Autodesk Inventor part; units mm, degrees
ref_plane "YZ Plane" through (0, 0, 0) normal (1, 0, 0) x (0, 1, 0)
ref_plane "XZ Plane" through (0, 0, 0) normal (0, 1, 0) x (-1, 0, 0)
ref_plane "XY Plane" through (0, 0, 0) normal (0, 0, 1) x (1, 0, 0)
sketch "Sketch1" plane through (0, 0, 0) normal (0, 0, 1) x (1, 0, 0)
  line L0 (0, 18.05) -> (16, 18.05)
  line L1 (16, 18.05) -> (16, -18.05)
  line L2 (16, -18.05) -> (0, -18.05)
  arc A0 (0, -8.15) -> (0, 8.15) centre (0, 0) ccw
  line L3 (0, -18.05) -> (0, -8.15)
  line L4 (0, 8.15) -> (0, 18.05)
  point P0 (16, 0)
  dimension "d0" = 16.3
  dimension "d1" = 36.1
  dimension "d3" = 16
extrude "Extrusion1" add sketch "Sketch1" along normal mid plane 5
sketch "Sketch2" plane through (0, 0, 2.5) normal (0, 0, 1) x (1, 0, 0)
  arc A0 (0, -6.25) -> (0, 6.25) centre (0, 0) ccw
  arc A1 (0, -8.15) -> (0, 8.15) centre (0, 0) ccw
  line L0 (0, 6.25) -> (0, 8.15)
  line L1 (0, -6.25) -> (0, -8.15)
  dimension "d6" = 12.5
extrude "Extrusion2" add sketch "Sketch2" along normal blind 3.8 and the other way blind 1.8
sketch "Sketch3" plane through (0, 0, 6.3) normal (0, 0, 1) x (1, 0, 0)
  arc A0 (0, -8.15) -> (0, 8.15) centre (0, 0) ccw
  arc A1 (0, -11.15) -> (0, 11.15) centre (0, 0) ccw
  line L0 (0, -8.15) -> (0, -11.15)
  line L1 (0, 8.15) -> (0, 11.15)
  dimension "d11" = 3
extrude "Extrusion3" add sketch "Sketch3" along normal blind 4
sketch "Sketch4" plane through (0, 0, 6.3) normal (0, 0, -1) x (-1, 0, 0)
  arc A0 (0, 8.15) -> (0, -8.15) centre (0, 0) ccw
  line L0 (0, 11.15) -> (0, 8.15)
  arc A1 (0, 11.15) -> (0, -11.15) centre (0, 0) ccw
  line L1 (0, -8.15) -> (0, -11.15)
extrude "Extrusion4" add sketch "Sketch4" along normal up to surface (3.8 mm away)
sketch "Sketch5" plane through (0, 0, 2.5) normal (0, 0, 1) x (1, 0, 0)
  arc A0 (0, -11.15) -> (0, 11.15) centre (0, 0) ccw
  line L0 (16, 18.05) -> (0, 18.05)
  line L1 (3, 18.05) -> (3, 10.7388)
  arc A1 (0, -11.15) -> (0, 11.15) centre (0, 0) ccw
  line L2 (3, -10.7388) -> (3, -18.05)
  line L3 (0, -18.05) -> (16, -18.05)
  line L4 (0, 18.05) -> (0, 11.15)
  line L5 (0, -11.15) -> (0, -18.05)
  dimension "d16" = 3
extrude "Extrusion5" add sketch "Sketch5" along normal up to surface (7.8 mm away)
chamfer "Chamfer1" distance 5 angle 45 1 edges at (11.15, 0, 2.5)
fillet "Fillet1" radius 3 3 edges at (11.7041, -11.1281, 2.5) (11.15, 0, 7.5) (11.7041, 11.1281, 2.5)
sketch "Sketch6" plane through (3, -18.05, 2.5) normal (1, 0, 0) x (0, 0, -1)
  circle A0 centre (-3.8, 32.1) radius 1.6
  circle A1 centre (-3.8, 4) radius 1.6
  line L0 (0, 0) -> (-7.8, 0)
  line L1 (-7.8, 7.3112) -> (-7.8, 0)
  line L2 (0, 36.1) -> (-7.8, 36.1)
  point P0 (2.5, 18.05)
  dimension "d19" = 3.2
  dimension "d20" = 4
  dimension "d21" = 4
  dimension "d22" = 4
extrude "Extrusion6" cut sketch "Sketch6" against normal up to next
fillet "Fillet2" radius 4 2 edges at (1.5, -18.05, 10.3) (1.5, 18.05, 10.3)
fillet "Fillet3" radius 4 2 edges at (16, -18.05, 0) (16, 18.05, 0)
sketch "Sketch7" plane through (3, -18.05, 2.5) normal (1, 0, 0) x (0, 0, -1)
  arc A0 (-3.2482, 5.5018) -> (-2.2844, 4.5129) centre (-3.8, 4) ccw
  arc A1 (-2.2844, 31.5871) -> (-3.2482, 30.5982) centre (-3.8, 32.1) ccw
  circle A2 centre (-3.8, 4) radius 3.5
  circle A3 centre (-3.8, 32.1) radius 3.5
  point P0 (2.5, 18.05)
  dimension "d31" = 7
extrude "Extrusion7" cut sketch "Sketch7" along normal through all
properties part number "x-carriage-holder"
Read the model definition and answer for the solid it produces. Units are mm, in the model's axes. A direction names the side the tool comes from. Give positions to 0.01 mm unless a question says otherwise; leave off trailing zeros. Write each loop counter-clockwise with the first axis right and the second up, starting at its lowest first coordinate (ties: lowest second). Pieces come first, ordered by that corner, then holes. Notation, with made-up numbers: (36, -11) - (80, -11) arc R8 cw to (80, -6) - close; hole circle Ø7 at (30, 62). An arc over 180 degrees is marked (long way). Return JSON: item names as keys, results as strings.
Q1. For a pull along Y with two mould halves and no side action, classify faces 6 (the face through (12, -15, 2.5)), 7 (the face through (1, 17, 9)), 8 (the face through (5.4, -11.5, 3.9)), 9 (the face through (6.25, 0.14, 3.46)) as released by +Y, released by -Y, zero draft, split by the parting line, or undercut.
Reply:
{"face 6": "zero draft", "face 7": "released by +Y", "face 8": "undercut", "face 9": "undercut"}
Q2. A cutting plane is placed at C-C, the plane x = 2.5. Determine the outline of the cut face in (y, z).
Reply:
{"outline": "(-18.05, -2.5) - (-7.76, -2.5) - (-7.76, 0.7) - (-5.73, 0.7) - (-5.73, 6.3) - (-7.76, 6.3) - (-7.76, 10.3) - (-14.05, 10.3) arc R4 ccw to (-18.05, 6.3) - close; (5.73, 0.7) - (7.76, 0.7) - (7.76, -2.5) - (18.05, -2.5) - (18.05, 6.3) arc R4 ccw to (14.05, 10.3) - (7.76, 10.3) - (7.76, 6.3) - (5.73, 6.3) - close; hole circle Ø3.2 at (-14.05, 6.3); hole circle Ø3.2 at (14.05, 6.3)"}
Q3. A cutting plane is placed at D-D, the plane z = 2. Determine the outline of the cut face in (x, y), and give its area (3 significant figures).
Reply:
{"outline": "(0, -18.05) - (12, -18.05) arc R4 ccw to (16, -14.05) - (16, 14.05) arc R4 ccw to (12, 18.05) - (0, 18.05) - (0, 6.25) arc R6.25 cw to (0, -6.25) - close", "area": "509 mm²"}
Q4. Consider line 1 along Z through (x, y) = (1.3, -14.05); line 2 along Y through (x, z) = (4, 0.75); line 3 along X through (y, z) = (11.5, 4). Determine where each line is inside the solid, lowest interval first. Write a range as [from, to].
Reply:
{"line 1": "[-2.5, 4.7], [7.9, 10.3]", "line 2": "[-18.05, -4.8], [4.8, 18.05]", "line 3": "[0, 3]"}
Q5. A cutting plane is placed at B-B, the plane y = 0. Determine the outline of the cut face in (x, z), and give its area (3 significant figures).
Reply:
{"outline": "(6.25, 0.7) - (8.15, 0.7) - (8.15, -2.5) - (16, -2.5) - (16, 2.84) arc R3 cw to (15.27, 3.38) - (12.03, 6.62) arc R3 cw to (11.15, 8.74) - (11.15, 10.3) - (8.15, 10.3) - (8.15, 6.3) - (6.25, 6.3) - close", "area": "86.0 mm²"}
Q6. A cutting plane is placed at A-A, the plane z = 7. Determine the outline of the cut face in (x, y), and give its area (3 significant figures).
Reply:
{"outline": "(0, -17.99) - (3, -17.99) - (3, -15.49) - (0, -15.49) - close; (0, -12.61) - (3, -12.61) - (3, -10.62) - (4.93, -10.62) arc R11.71 ccw to (4.93, 10.62) - (3, 10.62) - (3, 12.61) - (0, 12.61) - (0, 8.15) arc R8.15 cw to (0, -8.15) - close; (0, 15.49) - (3, 15.49) - (3, 17.99) - (0, 17.99) - close", "area": "131 mm²"}
Q7. Given P1, Ø3.5, axis at x = 7, y = 15, coming from the +Z side; P2, Ø3.5, axis at x = 12.5, y = -11.5, coming from the +Z side; P3, Ø5, axis at x = 13.5, y = -6.5, coming from the +Z side; P4, Ø2.5, axis at y = 14.05, z = 6.3, coming from the -X side, each flat-ended and moving along its own axis, determine where each tip first touches the part or whether it passes through.
Reply:
{"P1": "z = 2.92", "P2": "z = 3.41", "P3": "z = 6.17", "P4": "through"}
Q8. For faces 1 (the face through (11.15, -0.2, 9.53)), 2 (the face through (8.15, 0.18, 8.27)), 3 (the face through (12, 15, 2.5)), 4 (the face through (8.15, 0.18, -0.92)), 5 (the face through (5, -18.05, 1)), determine the directions among +Z, -Z, +X, -X, +Y, -Y from which every point of the face is accessible in a straight line to the end or side of a thin tool.
Reply:
{"face 1": "+Z, +X", "face 2": "+Z, -X", "face 3": "+Z, +X, +Y", "face 4": "-Z, -X", "face 5": "+Z, -Z, +X, -X, -Y"}
